Geometry: final body of the model. Coordinates: model frame, mm. Face numbers are marked on the shaded views. A direction names the side the tool comes from. Give positions to 0.01 mm unless a question says otherwise; leave off trailing zeros. Order: outer loops, then holes, each group sorted by start corner. A loop starts at its lowest first (then second) coordinate and runs counter-clockwise, first axis right, second up. Notation, with made-up numbers: M 70.5,28 L 94.5,28 A13 cw 94.5,44 Z; hole C 51.25,-23 d8. An arc over 180 degrees is marked long. One line per item, written item: value. Start each with the question number.
```python
from build123d import *

# Parameters (mm, degrees)
SKETCH1_W                    = 38.1
SKETCH1_H                    = 38.1
MAIN_BODY_DEPTH              = 34
F_9_32_RIGHT_RAIL_DEPTH      = 64.712008287
F_9_32_RIGHT_RAIL_DEPTH_BACK = 5.55625
SKETCH3_R                    = 3.571875
SKETCH4_R                    = 3.571875
F_9_32_LEFT_RAIL_DEPTH       = 5.55625
F_9_32_TOPPER_DEPTH          = 64.712008287
F_9_32_TOPPER_DEPTH_BACK     = 10
SKETCH8_R                    = 3.571875
HEX_START                    = -5.55625
HEX_HOLE_RIGHT_DEPTH         = 32.54375
HEX_HOLE_LEFT_DEPTH          = 32.54375
INNER_START                  = -34
INNER_CAVITY_OUTLINE_W       = 26.9875
INNER_CAVITY_OUTLINE_H       = 26.9875
INNER_CAVITY_DEPTH           = 25.26875
HEX_START_2                  = -17
HEX_HOLE_TOP_DEPTH           = 13.825
TOP_CORNER_REACH             = 65.712


# Read off the part's stored shape, not the designer's step: Inner Cavity
with BuildPart() as part:
    # Sketch1 → Main Body (new body)
    with BuildSketch(Plane(origin=(0, 0, 0), x_dir=(1, 0, 0), z_dir=(0, 1, 0))):
        with Locations((19.05, 19.05)):
            Rectangle(SKETCH1_W, SKETCH1_H)
    extrude(amount=MAIN_BODY_DEPTH)

    # Sketch3 → 9/32 Right Rail (cut, two sides: drawn at the far end of the back side and taken through both)
    with BuildSketch(Plane.XY.offset(-F_9_32_RIGHT_RAIL_DEPTH_BACK)):
        with Locations(Location((19.05, 17, 0), (0, 0, 180))):
            Circle(SKETCH3_R)
    extrude(amount=F_9_32_RIGHT_RAIL_DEPTH + F_9_32_RIGHT_RAIL_DEPTH_BACK, mode=Mode.SUBTRACT)

    # Sketch4 → 9/32 Left Rail (cut)
    with BuildSketch(Plane.ZY):
        with Locations((-19.05, 17)):
            Circle(SKETCH4_R)
    extrude(amount=-F_9_32_LEFT_RAIL_DEPTH, mode=Mode.SUBTRACT)

    # Sketch8 → 9/32 Topper (cut, two sides: drawn at the far end of the back side and taken through both)
    with BuildSketch(Plane(origin=(0, 34, 0), x_dir=(1, 0, 0), z_dir=(0, 1, 0)).offset(-F_9_32_TOPPER_DEPTH_BACK)):
        with Locations(Location((19.05, 19.05, 0), (0, 0, 90))):
            Circle(SKETCH8_R)
    extrude(amount=F_9_32_TOPPER_DEPTH + F_9_32_TOPPER_DEPTH_BACK, mode=Mode.SUBTRACT)

    # Sketch9 → Hex Hole Right (cut)
    with BuildSketch(Plane.ZY.offset(HEX_START)):
        Polygon((-22.315182739, 22.6554624), (-25.580365478, 17), (-22.315182739, 11.3445376), (-15.784817261, 11.3445376), (-12.519634522, 17), (-15.784817261, 22.6554624), align=None)
    extrude(amount=-HEX_HOLE_RIGHT_DEPTH, mode=Mode.SUBTRACT)

    # Sketch10 → Hex Hole Left (cut)
    with BuildSketch(Plane.XY.offset(HEX_START)):
        Polygon((15.784813595, 22.65546875), (12.51962719, 17), (15.784813595, 11.34453125), (22.315186405, 11.34453125), (25.58037281, 17), (22.315186405, 22.65546875), align=None)
    extrude(amount=-HEX_HOLE_LEFT_DEPTH, mode=Mode.SUBTRACT)

    # Inner Cavity outline → Inner Cavity (cut)
    with BuildSketch(Plane(origin=(0, 34, 0), x_dir=(1, 0, 0), z_dir=(0, 1, 0)).offset(INNER_START)):
        with Locations((24.60625, 24.60625)):
            Rectangle(INNER_CAVITY_OUTLINE_W, INNER_CAVITY_OUTLINE_H)
    extrude(amount=INNER_CAVITY_DEPTH, mode=Mode.SUBTRACT)

    # Sketch14 → Hex Hole Top (cut)
    with BuildSketch(Plane(origin=(0, 34, 0), x_dir=(1, 0, 0), z_dir=(0, 1, 0)).offset(HEX_START_2)):
        Polygon((24.70546875, 22.315186405), (19.05, 25.58037281), (13.39453125, 22.315186405), (13.39453125, 15.784813595), (19.05, 12.51962719), (24.70546875, 15.784813595), align=None)
    extrude(amount=HEX_HOLE_TOP_DEPTH, mode=Mode.SUBTRACT)

    # Sketch16 → Top Corner (cut, up to next)
    with BuildSketch(Plane(origin=(0, 34, 0), x_dir=(1, 0, 0), z_dir=(0, 1, 0)), mode=Mode.PRIVATE) as top_corner_sk1:
        Polygon((38.1, 38.1), (16.276714219, 38.1), (38.1, 16.276714219), align=None)
    top_corner_tool1 = extrude(top_corner_sk1.sketch, amount=-TOP_CORNER_REACH, mode=Mode.PRIVATE) & part.part
    add(top_corner_tool1.solids().sort_by_distance((30.825571, 34, -30.825571))[0], mode=Mode.SUBTRACT)


solid = part.part
```
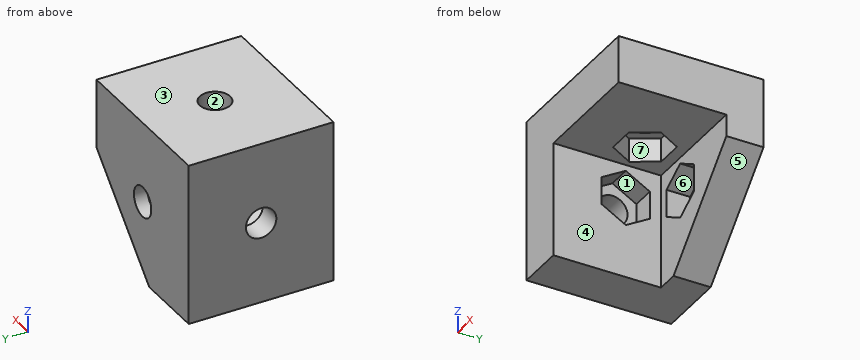
Q1. Section query C-C on z = -19.05. Return loops of the section in (x, y) (1 decimal).
Q2. Set-up query: the marked faces 4, 5, 6 and 7. Return all of +Z, -Z, +X, -X, +Y, -Y with unobstructed straight access to the full face (end or side cutting, diameter ignored); none if empty.
Q3. Contact query for flat-ended pins moving along their axis: pin 1 (10 mm diameter, centred on y = 22, z = -32, fed in from +X); pin 2 (3.5 mm diameter, centred on x = 21, y = 17.5, fed in from -Z); pin 3 (8 mm diameter, centred on x = 30, z = -21.5, fed in from -Y); pin 4 (5.5 mm diameter, centred on y = 17, z = -19.05, fed in from -X) (1 decimal). Output: stop coordinate, or through.
Q4. Section query D-D on x = 21. Return loops of the section in (y, z) (1 decimal), and give its area (3 significant figures).
Q5. Section query A-A on z = -9. Return loops of the section in (x, y).
Q6. Section query B-B on y = 28. Return loops of the section in (x, z).
Q7. Mould query, pull axis Z, two halves, no side actions, for the marked faces 1, 2 and 3. Classes: +Z half, -Z half, draft (parallel to the pull), parting line (faces both ways), or undercut.
Q8. Ray query, line 1 along Z through (x, y) = (10, 17); line 2 along X through (y, z) = (17, -4); line 3 along Y through (x, z) = (1.2, -19.05). Return the intervals inside material, ascending. Write a range as [from, to].
Results below:
1. outline: M 0,0 L 11.1,0 L 11.1,11.3 L 5.6,11.3 L 5.6,13.4 L 0,13.4 Z; M 0,20.6 L 5.6,20.6 L 5.6,22.7 L 11.1,22.7 L 11.1,25.3 L 13.4,25.3 L 13.4,30.8 L 15.5,30.8 L 15.5,34 L 0,34 Z; M 22.6,30.8 L 24.7,30.8 L 24.7,25.3 L 35.3,25.3 L 35.3,34 L 22.6,34 Z
2. face 4: -Z, +X, -Y
2. face 5: -Z, +X, +Y, -Y
2. face 6: -Y
2. face 7: -Z
3. pin 1: x = 26.16
3. pin 2: z = -5.56
3. pin 3: y = 25.27
3. pin 4: through
4. outline: M 0,-11.1 L 11.3,-11.1 L 11.3,-5.6 L 14,-5.6 L 14,0 L 0,0 Z; M 20,-5.6 L 22.7,-5.6 L 22.7,-11.1 L 25.3,-11.1 L 25.3,-13.6 L 30.8,-13.6 L 30.8,-16.1 L 34,-16.1 L 34,0 L 20,0 Z; M 25.3,-33.4 L 34,-33.4 L 34,-22 L 30.8,-22 L 30.8,-24.5 L 25.3,-24.5 Z
4. area: 397 mm2
5. outline: M 0,0 L 38.1,0 L 38.1,34 L 0,34 Z; hole M 12.52,17 L 15.78,11.34 L 22.32,11.34 L 25.58,17 L 22.32,22.66 L 15.78,22.66 Z
6. outline: M 0,-38.1 L 16.28,-38.1 L 38.1,-16.28 L 38.1,0 L 0,0 Z; hole M 13.39,-22.32 L 19.05,-25.58 L 24.71,-22.32 L 24.71,-15.78 L 19.05,-12.52 L 13.39,-15.78 Z
7. face 1: undercut
7. face 2: draft
7. face 3: +Z half
8. line 1: [-38.1, -25.58], [-12.52, 0]
8. line 2: [0, 15.48], [22.62, 38.1]
8. line 3: [0, 13.43], [20.57, 34]
